The listing builds one solid part. Answer for the finished solid, in the listing's coordinates (mm). Face numbers are marked on the shaded views. A direction names the side the tool comes from. Coordinates: 2 decimals unless noted, no trailing zeros. Order: outer loops, then holes, each group sorted by start corner. A loop starts at its lowest first (then second) coordinate and runs counter-clockwise, first axis right, second up. Notation, with made-up numbers: (40, 16.5) -> (96, 16.5) arc R17 ccw to (96, 39.5) -> close; hole circle Ø7 at (-34, -26). An arc over 180 degrees is marked (long way). Return JSON: item names as keys, results as strings.
```python
from build123d import *

# Parameters (mm, degrees)
SKETCH1_R               = 15.875
SKETCH1_R_2             = 9.525
BOSS_EXTRUDE1_DEPTH     = 12.7
SKETCH10_R              = 1.7272
CUT_EXTRUDE3_DEPTH      = 12.7
SKETCH5_R               = 1.7272
CUT_EXTRUDE4_DEPTH      = 12.7
BOSS_EXTRUDE6_DEPTH     = 6.35
SKETCH1_9_W             = 9.525
SKETCH1_9_H             = 31.75
BOSS_EXTRUDE7_DEPTH     = 25.4
RIB18_START             = -3.175
RIB18_DEPTH             = 6.35
CUT_EXTRUDE5_DEPTH      = 8.001
BOSS_EXTRUDE8_DEPTH     = 9.525
BOSS_EXTRUDE9_DEPTH     = 11.176
CUT_EXTRUDE6_DEPTH      = 44.196
CUT_EXTRUDE6_DEPTH_BACK = 50.8
SKETCH22_R              = 1.7272


with BuildPart() as part:
    # Sketch1 → Boss-Extrude1 (new body)
    with BuildSketch(Plane(origin=(0, 0, 0), x_dir=(1, 0, 0), z_dir=(0, 1, 0))):
        with Locations(Location((0, 0, 0), (0, 0, 270))):
            Circle(SKETCH1_R)
        with Locations(Location((0, 0, 0), (0, 0, 270))):
            Circle(SKETCH1_R_2, mode=Mode.SUBTRACT)
    extrude(amount=BOSS_EXTRUDE1_DEPTH)

    # Sketch10 → Cut-Extrude3 (cut)
    with BuildSketch(Plane(origin=(-11.225320151, 0, -11.225320151), x_dir=(-0.7071067811865486, 0, 0.7071067811865465), z_dir=(-0.7071067811865465, 0, -0.7071067811865486))):
        with Locations((0, 7.874)):
            Circle(SKETCH10_R)
    extrude(amount=-CUT_EXTRUDE3_DEPTH, mode=Mode.SUBTRACT)

    # Sketch5 → Cut-Extrude4 (cut)
    with BuildSketch(Plane(origin=(-11.225320151, 0, 11.225320151), x_dir=(0.7071067811865488, 0, 0.7071067811865464), z_dir=(-0.7071067811865464, 0, 0.7071067811865488))):
        with Locations((0, 7.874)):
            Circle(SKETCH5_R)
    extrude(amount=-CUT_EXTRUDE4_DEPTH, mode=Mode.SUBTRACT)

    # Sketch1<8> → Boss-Extrude6 (add)
    with BuildSketch(Plane(origin=(0, 0, 0), x_dir=(1, 0, 0), z_dir=(0, 1, 0))):
        with BuildLine():
            Line((0, -15.875), (15.875, -15.875))
            Line((15.875, -15.875), (15.875, 0))
            ThreePointArc((15.875, 0), (11.225320151, -11.225320151), (0, -15.875))
        make_face()
        with BuildLine():
            Line((15.875, 0), (15.875, 15.875))
            Line((15.875, 15.875), (0, 15.875))
            ThreePointArc((0, 15.875), (11.225320151, 11.225320151), (15.875, 0))
        make_face()
        Polygon((44.45, -15.875), (44.45, 15.875), (15.875, 15.875), (15.875, 0), (15.875, -15.875), align=None)
    extrude(amount=BOSS_EXTRUDE6_DEPTH)

    # Sketch1<9> → Boss-Extrude7 (add)
    with BuildSketch(Plane(origin=(0, 0, 0), x_dir=(1, 0, 0), z_dir=(0, 1, 0))):
        with Locations((49.2125, 0)):
            Rectangle(SKETCH1_9_W, SKETCH1_9_H)
    extrude(amount=BOSS_EXTRUDE7_DEPTH)

    # Rib18: read off the stored shape, not the designer's step
    # Rib18 outline → Rib18 (add)
    with BuildSketch(Plane.XY.offset(RIB18_START)):
        with BuildLine():
            Line((15.847686346, 12.7), (15.554259867, 12.7))
            Line((15.554259867, 12.7), (15.554259867, 6.35))
            Line((15.554259867, 6.35), (44.45, 6.35))
            Line((44.45, 6.35), (44.45, 25.4))
            Line((44.45, 25.4), (20.13457386, 11.562910878))
            ThreePointArc((20.13457386, 11.562910878), (18.809330508, 11.231428329), (17.504040967, 11.634379737))
            Line((17.504040967, 11.634379737), (15.847686346, 12.7))
        make_face()
    extrude(amount=RIB18_DEPTH)

    # Sketch20 → Cut-Extrude5 (cut)
    with BuildSketch(Plane(origin=(53.975, 0, 0), x_dir=(0, 0, -1), z_dir=(1, 0, 0))):
        with BuildLine():
            ThreePointArc((-10.3378, 6.35), (-10.876615367, 6.573184633), (-11.0998, 7.112))
            Line((-11.0998, 7.112), (-11.0998, 11.938))
            ThreePointArc((-11.0998, 11.938), (-10.876615367, 12.476815367), (-10.3378, 12.7))
            Line((-10.3378, 12.7), (10.3378, 12.7))
            ThreePointArc((10.3378, 12.7), (10.876615367, 12.476815367), (11.0998, 11.938))
            Line((11.0998, 11.938), (11.0998, 7.112))
            ThreePointArc((11.0998, 7.112), (10.876615367, 6.573184633), (10.3378, 6.35))
            Line((10.3378, 6.35), (-10.3378, 6.35))
        make_face()
    extrude(amount=-CUT_EXTRUDE5_DEPTH, mode=Mode.SUBTRACT)

    # Sketch20<3> → Boss-Extrude8 (add)
    with BuildSketch(Plane(origin=(53.975, 0, 0), x_dir=(0, 0, -1), z_dir=(1, 0, 0))):
        with BuildLine():
            Line((-15.875, 25.4), (-9.525, 25.4))
            ThreePointArc((-9.525, 25.4), (0, 34.925), (9.525, 25.4))
            Line((9.525, 25.4), (15.875, 25.4))
            ThreePointArc((15.875, 25.4), (0, 41.275), (-15.875, 25.4))
        make_face()
        with BuildLine():
            ThreePointArc((9.525, 25.4), (0, 34.925), (-9.525, 25.4))
            Line((-9.525, 25.4), (9.525, 25.4))
        make_face()
        with BuildLine():
            Line((9.525, 25.4), (-9.525, 25.4))
            ThreePointArc((-9.525, 25.4), (0, 15.875), (9.525, 25.4))
        make_face()
    extrude(amount=-BOSS_EXTRUDE8_DEPTH)

    # Sketch20<4> → Boss-Extrude9 (add)
    with BuildSketch(Plane(origin=(53.975, 0, 0), x_dir=(0, 0, -1), z_dir=(1, 0, 0))):
        with BuildLine():
            ThreePointArc((9.525, 25.4), (0, 34.925), (-9.525, 25.4))
            Line((-9.525, 25.4), (9.525, 25.4))
        make_face()
        with BuildLine():
            Line((9.525, 25.4), (-9.525, 25.4))
            ThreePointArc((-9.525, 25.4), (0, 15.875), (9.525, 25.4))
        make_face()
    extrude(amount=BOSS_EXTRUDE9_DEPTH)

    # Sketch22 → Cut-Extrude6 (cut, two sides: drawn at the far end of the back side and taken through both)
    with BuildSketch(Plane.XY.offset(-CUT_EXTRUDE6_DEPTH_BACK)):
        with Locations(Location((50.8, 9.850914973, 0), (0, 0, 180))):
            Circle(SKETCH22_R)
    extrude(amount=CUT_EXTRUDE6_DEPTH + CUT_EXTRUDE6_DEPTH_BACK, mode=Mode.SUBTRACT)


solid = part.part
```
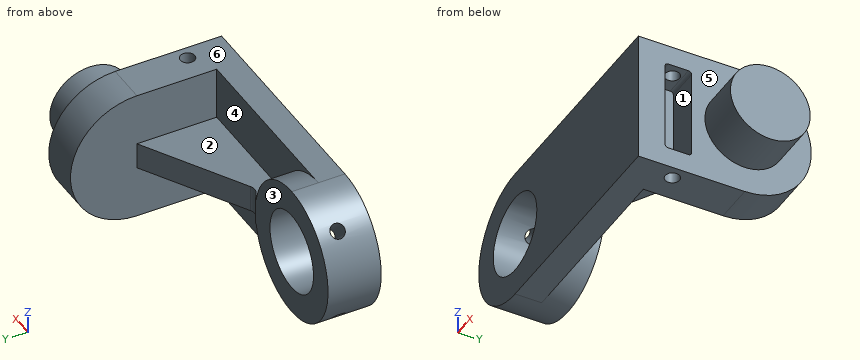
Item 1: Find the intervals of material crossed by probe 1 along X at (y, z) = (7, 0) (3 decimals); probe 2 along Z at (x, y) = (31, 8) (3 decimals); probe 3 along X at (y, z) = (37.5, -7) (3 decimals), in increasing order.
Answer list:
{"probe 1": "-15.875 to -9.525, 9.525 to 45.974", "probe 2": "-3.175 to 3.175", "probe 3": "44.45 to 53.975"}
Item 2: The part is cut by section D-D on x = -3. Determine the outline of the cut face in (y, z).
Answer list:
{"outline": "(0, -15.59) -> (12.7, -15.59) -> (12.7, -9.04) -> (0, -9.04) -> close; (0, 9.04) -> (12.7, 9.04) -> (12.7, 15.59) -> (0, 15.59) -> close"}
Item 3: The part is cut by section B-B on x = 50.8. Determine the outline of the cut face in (y, z) (3 decimals).
Answer list:
{"outline": "(0, -15.875) -> (8.124, -15.875) -> (8.124, -11.1) -> (7.112, -11.1) arc R0.762 cw to (6.35, -10.338) -> (6.35, 10.338) arc R0.762 cw to (7.112, 11.1) -> (8.124, 11.1) -> (8.124, 15.875) -> (0, 15.875) -> close; (11.578, -15.875) -> (25.4, -15.875) arc R15.875 ccw to (25.4, 15.875) -> (11.578, 15.875) -> (11.578, 11.1) -> (11.938, 11.1) arc R0.762 cw to (12.7, 10.338) -> (12.7, -10.338) arc R0.762 cw to (11.938, -11.1) -> (11.578, -11.1) -> close"}
Item 4: The part is cut by section C-C on y = 31. Determine the outline of the cut face in (x, z) (3 decimals).
Answer list:
{"outline": "(44.45, -14.854) -> (53.975, -14.854) -> (53.975, -7.705) -> (65.151, -7.705) -> (65.151, 7.705) -> (53.975, 7.705) -> (53.975, 14.854) -> (44.45, 14.854) -> close"}
Item 5: Determine the mould class of the marked faces 4, 5 and 6 for opening direction X: pulls with the +X half, pulls with the -X half, needs draft (parallel to the pull), parting line crosses it, or undercut.
Answer list:
{"face 4": "undercut", "face 5": "pulls with the +X half", "face 6": "needs draft"}
Item 6: Which of the six approach directions +Z, -Z, +X, -X, +Y, -Y give full straight-line access (tool end or side, diameter ignored) to the marked faces 1, 2 and 3?
Answer list:
{"face 1": "+X", "face 2": "+Z, +Y", "face 3": "+Z, -Z, -X, +Y"}
Item 7: Flat-ended cylindrical pins translate along their axes: pin 1 (21 mm diameter, centred on x = 25, y = 19, fed in from +Z) (3 decimals); pin 2 (15 mm diameter, centred on x = 36, y = 18.5, fed in from -Z) (3 decimals); pin 3 (7 mm diameter, centred on y = 11, z = 1.5, fed in from +X) (3 decimals). Find the tip coordinate at first contact, or state that the pin passes through.
Answer list:
{"pin 1": "z = 3.175", "pin 2": "z = -3.175", "pin 3": "x = 53.975"}
